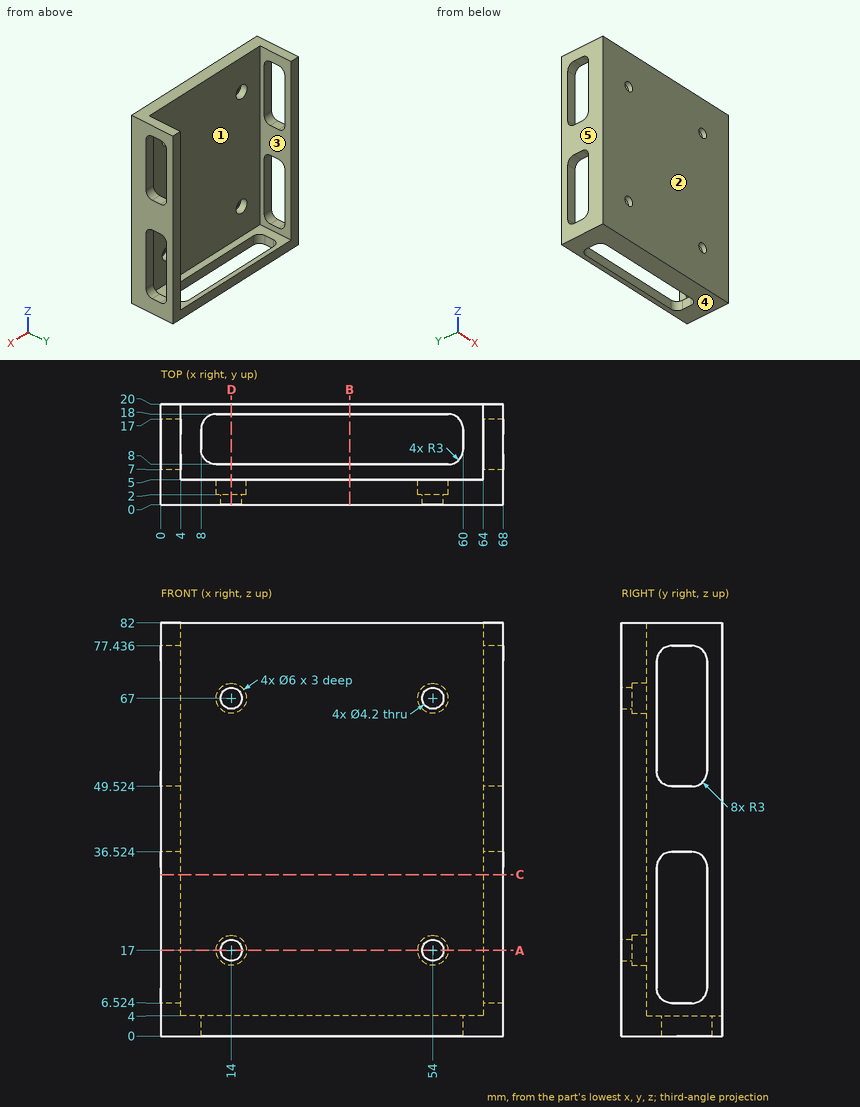
Job drawing, mm, ordinate dimensions from the low corner. One solid piece. A direction names the side the tool comes from. Give positions to 0.01 mm unless a question says otherwise; leave off trailing zeros. Order: outer loops, then holes, each group sorted by start corner. A loop starts at its lowest first (then second) coordinate and runs counter-clockwise, first axis right, second up. Notation, with made-up numbers: (80, -6.5) - (118, -6.5) arc R9 cw to (118, 9.5) - close; hole circle Ø1 at (13, 27.5). An arc over 180 degrees is marked (long way). Answer in a Markdown table with one row per item.
1. Saw through at B-B, the plane x = 37.5. Give the cut face in (y, z).
Data:
| item | result |
|---|---|
| outline | (0, 0) - (8, 0) - (8, 4) - (5, 4) - (5, 82) - (0, 82) - close; (18, 0) - (20, 0) - (20, 4) - (18, 4) - close |
2. Tool access for the marked faces 1 and 2: list every direction of +Z, -Z, +X, -X, +Y, -Y with a clear straight run to the whole face (end or side of a thin tool).
Data:
| item | result |
|---|---|
| face 1 | +Z, +Y |
| face 2 | +Z, -Z, +X, -X, -Y |
3. Saw through at A-A, the plane z = 17. Count the separate pieces of the cut face and the enclosed holes in it, plus the area to 3 significant figures.
Data:
| item | result |
|---|---|
| separate pieces | 5 |
| enclosed holes | 0 |
| area | 327 mm² |
4. Flat gauge pins, fed straight in: pin 1 (5 mm diameter, centred on y = 11, z = 16.5, fed in from -X); pin 2 (8 mm diameter, centred on x = 54, z = 67, fed in from +Y); pin 3 (8 mm diameter, centred on x = 16, y = 11, fed in from +Z). Where does each tip first touch, or does it go through?
Data:
| item | result |
|---|---|
| pin 1 | passes through |
| pin 2 | stops at y = 5 |
| pin 3 | stops at z = 4 |
5. Saw through at C-C, the plane z = 32. Give the cut face in (x, y).
Data:
| item | result |
|---|---|
| outline | (0, 0) - (68, 0) - (68, 7) - (64, 7) - (64, 5) - (4, 5) - (4, 7) - (0, 7) - close; (0, 17) - (4, 17) - (4, 20) - (0, 20) - close; (64, 17) - (68, 17) - (68, 20) - (64, 20) - close |
6. Pull direction X, two halves, no side cores. Call the marked faces 3, 4 and 5: pulls with the +X half, pulls with the -X half, needs draft (parallel to the pull), parting line crosses it, or undercut.
Data:
| item | result |
|---|---|
| face 3 | undercut |
| face 4 | needs draft |
| face 5 | pulls with the -X half |
7. Probe probe 1 along X at (y, z) = (0.95, 17); probe 2 along X at (y, z) = (4.3, 67); probe 3 along X at (y, z) = (8.25, 48). List the from-to ranges inside material, lowest first. Write a range as [from, to].
Data:
| item | result |
|---|---|
| probe 1 | x = [0, 11.9], [16.1, 51.9], [56.1, 68] |
| probe 2 | x = [0, 11], [17, 51], [57, 68] |
| probe 3 | x = [0, 4], [64, 68] |
8. Saw through at D-D, the plane x = 14. Give the cut face in (y, z), plus the area to 3 significant figures.
Data:
| item | result |
|---|---|
| outline | (0, 0) - (8, 0) - (8, 4) - (5, 4) - (5, 14) - (2, 14) - (2, 14.9) - (0, 14.9) - close; (0, 19.1) - (2, 19.1) - (2, 20) - (5, 20) - (5, 64) - (2, 64) - (2, 64.9) - (0, 64.9) - close; (0, 69.1) - (2, 69.1) - (2, 70) - (5, 70) - (5, 82) - (0, 82) - close; (18, 0) - (20, 0) - (20, 4) - (18, 4) - close |
| area | 377 mm² |
